Read the model definition and answer for the solid it produces. Units are mm, in the model's axes. Face numbers are marked on the shaded views. Give positions to 0.01 mm unless a question says otherwise; leave off trailing zeros. Loops run counter-clockwise (first coordinate to the right, second up) from the corner with the lowest first, then second, coordinate; pieces in that order, holes last. Notation, with made-up numbers: (28.5, 18) -> (42.5, 18) arc R8 ccw to (42.5, 23) -> close; hole circle Ø3 at (9, -6.5). An arc over 180 degrees is marked (long way). Answer as CSV lines item,"result". Start each with the question number.
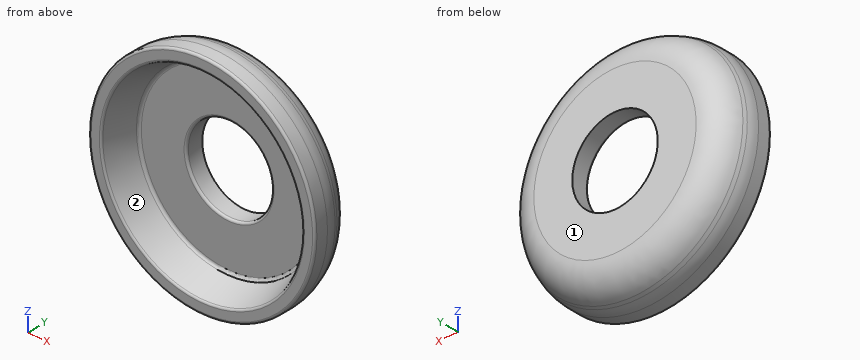
```python
from build123d import *


with BuildPart() as part:
    # Sketch1 → Revolve1 (revolve)
    with BuildSketch(Plane.XY):
        with BuildLine():
            Line((4.75, 4.25), (9.016237468, 4.25))
            ThreePointArc((9.016237468, 4.25), (10.973568282, 3.628502604), (12.213835367, 1.991694585))
            Line((12.213835367, 1.991694585), (12.352608297, 1.600607236))
            ThreePointArc((12.352608297, 1.600607236), (12.505509699, 1.015806617), (12.55697426, 0.413542553))
            Line((12.55697426, 0.413542553), (12.55697426, -0.91549471))
            ThreePointArc((12.55697426, -0.91549471), (12.483750956, -1.092271405), (12.30697426, -1.16549471))
            Line((12.30697426, -1.16549471), (11.388512384, -1.16549471))
            ThreePointArc((11.388512384, -1.16549471), (11.2442914, -1.119701242), (11.152905448, -0.999097171))
            Line((11.152905448, -0.999097171), (10.083602461, 2.014393064))
            ThreePointArc((10.083602461, 2.014393064), (9.954206532, 2.185159746), (9.75, 2.25))
            Line((9.75, 2.25), (5, 2.25))
            ThreePointArc((5, 2.25), (4.823223305, 2.323223305), (4.75, 2.5))
            Line((4.75, 2.5), (4.75, 4.25))
        make_face()
    revolve(axis=Axis((0, -4.993282938, 0), (0, 1, 0)))


solid = part.part
```
(1) Each of these flat-tipped pins is pushed along its axis until it touches: P1, Ø1, axis at y = 2, z = -7, coming from the -X side; P2, Ø2, axis at y = 1.5, z = 6, coming from the -X side; P3, Ø10, axis at x = 4, z = 1, coming from the -Y side; P4, Ø8, axis at x = -8.5, z = 1.5, coming from the -Y side. Where does it stop, or does it pass through?
(2) Find the intervals of material crossed by line 1 along Z through (x, y) = (7.75, -0.8); line 2 along Y through (x, z) = (4.25, -7.5); line 3 along Z through (x, y) = (0, 3.5), in increasing order. Write a range as from..to.
(3) Find section C-C on y = 3. Write down the section's boundary in (x, z), then the cut area to 3 significant figures.
(4) Find section A-A on z = 0. Write down the section's boundary in (x, y).
(5) The mould has two halves that part along X. Classify the marked faces 1 and 2: pulls with the +X half, pulls with the -X half, needs draft (parallel to the pull), parting line crosses it, or undercut.
(6) Find section B-B on x = 0. Write down the section's boundary in (y, z).
Answer block:
1,P1,"stops at x = -10.4"
1,P2,"stops at x = -11.41"
1,P3,"stops at y = 2.25"
1,P4,"stops at y = -1.17"
2,line 1,"z = -9.88..-7.92, 7.92..9.88"
2,line 2,"y = 2.25..4.25"
2,line 3,"z = -11.14..-4.75, 4.75..11.14"
3,outline,"circle Ø23.29 at (0, 0); hole circle Ø9.5 at (0, 0)"
3,area,"355 mm2"
4,outline,"(-12.56, -0.92) arc R0.25 ccw to (-12.31, -1.17) -> (-11.39, -1.17) arc R0.25 ccw to (-11.15, -1) -> (-10.08, 2.01) arc R0.35 cw to (-9.75, 2.25) -> (-5, 2.25) arc R0.25 ccw to (-4.75, 2.5) -> (-4.75, 4.25) -> (-9.02, 4.25) arc R3.39 ccw to (-12.21, 1.99) -> (-12.35, 1.6) arc R3.55 ccw to (-12.56, 0.41) -> close; (4.75, 2.5) arc R0.25 ccw to (5, 2.25) -> (9.75, 2.25) arc R0.35 cw to (10.08, 2.01) -> (11.15, -1) arc R0.25 ccw to (11.39, -1.17) -> (12.31, -1.17) arc R0.25 ccw to (12.56, -0.92) -> (12.56, 0.41) arc R3.55 ccw to (12.35, 1.6) -> (12.21, 1.99) arc R3.39 ccw to (9.02, 4.25) -> (4.75, 4.25) -> close"
5,face 1,"needs draft"
5,face 2,"undercut"
6,outline,"(-1.17, -12.31) arc R0.25 ccw to (-0.92, -12.56) -> (0.41, -12.56) arc R3.55 ccw to (1.6, -12.35) -> (1.99, -12.21) arc R3.39 ccw to (4.25, -9.02) -> (4.25, -4.75) -> (2.5, -4.75) arc R0.25 ccw to (2.25, -5) -> (2.25, -9.75) arc R0.35 cw to (2.01, -10.08) -> (-1, -11.15) arc R0.25 ccw to (-1.17, -11.39) -> close; (-1.17, 11.39) arc R0.25 ccw to (-1, 11.15) -> (2.01, 10.08) arc R0.35 cw to (2.25, 9.75) -> (2.25, 5) arc R0.25 ccw to (2.5, 4.75) -> (4.25, 4.75) -> (4.25, 9.02) arc R3.39 ccw to (1.99, 12.21) -> (1.6, 12.35) arc R3.55 ccw to (0.41, 12.56) -> (-0.92, 12.56) arc R0.25 ccw to (-1.17, 12.31) -> close"
